from build123d import *

# Parameters (mm, degrees)
F1_DEPTH = 63.5
F2_DEPTH = 25.4
F3_DEPTH = 7.9375
F5_R     = 6.35


with BuildPart() as f1:
    # F0 (on Front) → F1 (new body, symmetric)
    with BuildSketch(Plane.XZ):
        Polygon((41.275, -9.525), (41.275, 9.525), (22.225, 9.525), (-41.275, 9.525), (-41.275, -9.525), align=None)
    extrude(amount=F1_DEPTH, both=True)

    # F0 (on Front) → F2 (join, symmetric)
    with BuildSketch(Plane.XZ):
        with BuildLine():
            Line((22.225, 9.525), (41.275, 9.525))
            Line((41.275, 9.525), (41.275, 27.0002))
            ThreePointArc((41.275, 27.0002), (45.9246798487, 38.2255201513), (57.15, 42.8752))
            Line((57.15, 42.8752), (60.325, 42.8752))
            Line((60.325, 42.8752), (60.325, 61.9252))
            Line((60.325, 61.9252), (57.15, 61.9252))
            add(Edge.make_bspline(
                [(52.9513252364, 61.6718996299), (54.3293732693, 61.7682561346), (55.728666372, 61.8526413819), (57.15, 61.9252)],
                knots=[108.1713058896, 108.1713058896, 108.1713058896, 108.1713058896, 111.5045361635, 111.5045361635, 111.5045361635, 111.5045361635], degree=3))
            ThreePointArc((52.9513252364, 61.6718996299), (31.0119593206, 50.1639314446), (22.225, 27.0002))
            Line((22.225, 27.0002), (22.225, 9.525))
        make_face()
        Polygon((60.325, 61.9252), (60.325, 42.8752), (85.7630187815, 42.8752), (85.9146894524, 61.9252), align=None)
    extrude(amount=F2_DEPTH, both=True)

    # F0 (on Front) → F3 (join, symmetric)
    with BuildSketch(Plane.XZ):
        with BuildLine():
            Line((-41.275, 9.525), (22.225, 9.525))
            Line((22.225, 9.525), (22.225, 27.0002))
            ThreePointArc((22.225, 27.0002), (31.0119593206, 50.1639314446), (52.9513252364, 61.6718996299))
            add(Edge.make_bspline(
                [(-41.275, 9.525), (-14.1161793471, 42.8102760559), (8.2303659697, 58.5449002676), (52.9513252364, 61.6718996299)],
                knots=[0, 0, 0, 0, 108.1713058896, 108.1713058896, 108.1713058896, 108.1713058896], degree=3))
        make_face()
    extrude(amount=F3_DEPTH, both=True)

    # F0 (on Front) → F4 (revolve)
    with BuildSketch(Plane.XZ):
        Polygon((85.9146894524, 61.9252), (85.7630187815, 42.8752), (85.725, 38.1), (111.125, 38.1), (111.125, 66.675), (85.9525060063, 66.675), align=None)
    revolve(axis=Axis((85.8387530032, 0, 52.3875), (0.0079614627, 0, 0.9999683071)))

    # F5
    f5_edges = [f1.edges().sort_by_distance(p)[0] for p in [
        (41.275, 63.5, 0),
        (-41.275, 63.5, 0),
        (-41.275, -63.5, 0),
        (41.275, -63.5, 0),
    ]]
    fillet(f5_edges, radius=F5_R)


solid = f1.part
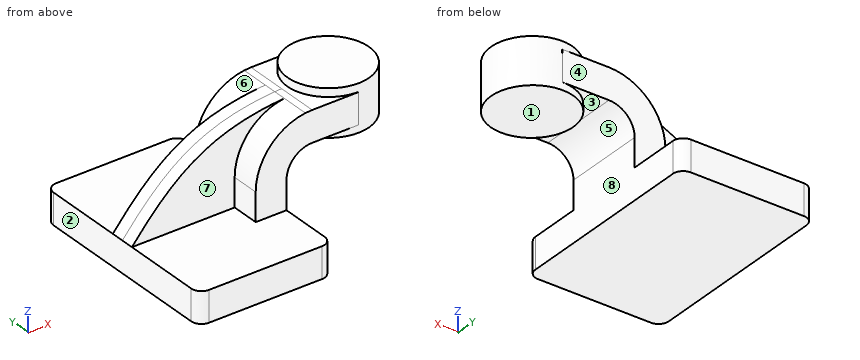
Geometry check sheet. Reference: the model listing, model coordinates, mm. Face numbers are marked on the shaded views. A direction names the side the tool comes from. Round coordinates to 2 decimals unless told otherwise and drop trailing zeros. Order: outer loops, then holes, each group sorted by start corner. A loop starts at its lowest first (then second) coordinate and runs counter-clockwise, first axis right, second up. Notation, with made-up numbers: M 36,38.25 L 59,38.25 A21 ccw 59,76.25 Z; hole C -38,47.25 d5. An arc over 180 degrees is marked long. Write each question's results on one line, items separated by ' | '. Start each with the question number.
1. Go/stop test with flat-tipped pins: P1, Ø5, axis at x = 41.5, y = 3.5, coming from the +Z side; P2, Ø16.5, axis at x = 6.5, y = -34.5, coming from the +Z side (3 decimals); P3, Ø3, axis at x = -13.5, z = 32.5, coming from the +Y side; P4, Ø2, axis at x = 59.5, z = 37, coming from the +Y side. Record where each tip stops, or that it passes through.
2. Draft check along X on the marked faces 1, 2, 3 and 4. Enter one of: pulls with the +X half, pulls with the -X half, needs draft (parallel to the pull), parting line crosses it, or undercut.
3. Set-up check for the marked faces 5, 6, 7 and 8: record each of +Z, -Z, +X, -X, +Y, -Y from which the full face is reachable in a straight line by a thin tool's end or side.
4. Cross-section at B-B on y = -37. Record the boundary of the cut face in (x, z) (3 decimals), plus the area to 3 significant figures.
5. Cross-section at A-A on z = 5. Record the boundary of the cut face in (x, y) (3 decimals), plus the area to 3 significant figures.
6. Material ranges on L1, parallel to Y at x = 50, z = 53; L2, parallel to Y at x = 18.5, z = 27; L3, parallel to Z at x = -6.5, y = 49.5 (3 decimals), recorded low to high. Write a range as from..to.
Resolved:
1) P1: z = 60.84 | P2: z = 9.525 | P3: y = 7.94 | P4: through
2) face 1: undercut | face 2: pulls with the -X half | face 3: undercut | face 4: needs draft
3) face 5: -Z, +Y, -Y | face 6: +Z, -X, +Y | face 7: +Z, -X, -Y | face 8: -Z, +X, +Y, -Y
4) outline: M -41.275,-9.525 L 41.275,-9.525 L 41.275,9.525 L -41.275,9.525 Z | area: 1,570 mm2
5) outline: M -41.275,-57.15 A6.35 ccw -34.925,-63.5 L 34.925,-63.5 A6.35 ccw 41.275,-57.15 L 41.275,57.15 A6.35 ccw 34.925,63.5 L -34.925,63.5 A6.35 ccw -41.275,57.15 Z | area: 10,400 mm2
6) L1: -25.4..25.4 | L2: -7.94..7.94 | L3: -9.525..9.525
